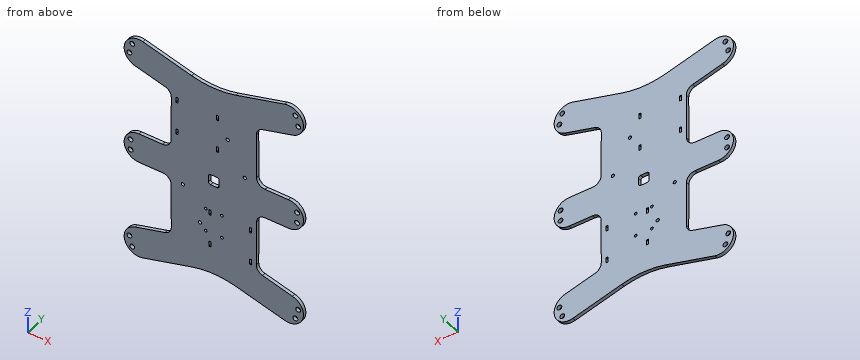
```python
from build123d import *

# Parameters (mm, degrees)
BOSS_EXTRUDE1_DEPTH = 3.175
FILLET1_R           = 80
FILLET2_R           = 8
SKETCH7_R           = 2.25
CUT_EXTRUDE4_DEPTH  = 10
CUT_EXTRUDE5_DEPTH  = 10
SKETCH9_W           = 10
SKETCH9_H           = 10
CUT_EXTRUDE6_DEPTH  = 10
FILLET3_R           = 2
SKETCH12_W          = 2
SKETCH12_H          = 5
CUT_EXTRUDE7_DEPTH  = 10
SKETCH13_R          = 1.25
CUT_EXTRUDE8_DEPTH  = 10


with BuildPart() as part:
    # Sketch1 → Boss-Extrude1 (new body)
    with BuildSketch(Plane(origin=(0, 0, 0), x_dir=(1, 0, 0), z_dir=(0, 1, 0))):
        with BuildLine():
            Line((-70, 14), (-40, 14))
            Line((-40, 14), (-39.816062711, 70))
            Line((-39.816062711, 70), (-73.623466631, 79.058666579))
            ThreePointArc((-73.623466631, 79.058666579), (-83.522961568, 96.205094778), (-66.376533369, 106.104589715))
            Line((-66.376533369, 106.104589715), (0, 88.319051202))
            Line((0, 88.319051202), (66.376533369, 106.104589715))
            ThreePointArc((66.376533369, 106.104589715), (83.522961568, 96.205094778), (73.623466631, 79.058666579))
            Line((73.623466631, 79.058666579), (39.816062711, 70))
            Line((39.816062711, 70), (40, 14))
            Line((40, 14), (70, 14))
            ThreePointArc((70, 14), (84, 0), (70, -14))
            Line((70, -14), (40, -14))
            Line((40, -14), (39.816062711, -70))
            Line((39.816062711, -70), (73.623466631, -79.058666579))
            ThreePointArc((73.623466631, -79.058666579), (83.522961568, -96.205094778), (66.376533369, -106.104589715))
            Line((66.376533369, -106.104589715), (0, -88.319051202))
            Line((0, -88.319051202), (-66.376533369, -106.104589715))
            ThreePointArc((-66.376533369, -106.104589715), (-83.522961568, -96.205094778), (-73.623466631, -79.058666579))
            Line((-73.623466631, -79.058666579), (-39.816062711, -70))
            Line((-39.816062711, -70), (-40, -14))
            Line((-40, -14), (-70, -14))
            ThreePointArc((-70, -14), (-84, 0), (-70, 14))
        make_face()
    extrude(amount=BOSS_EXTRUDE1_DEPTH)

    # Fillet1
    fillet1_edges = [part.edges().sort_by_distance(p)[0] for p in [
        (0, 1.5875, -88.319051202),
        (0, 1.5875, 88.319051202),
    ]]
    fillet(fillet1_edges, radius=FILLET1_R)

    # Fillet2
    fillet2_edges = [part.edges().sort_by_distance(p)[0] for p in [
        (-40, 1.5875, -14),
        (-39.816062711, 1.5875, -70),
        (39.816062711, 1.5875, -70),
        (40, 1.5875, -14),
        (40, 1.5875, 14),
        (39.816062711, 1.5875, 70),
        (-39.816062711, 1.5875, 70),
        (-40, 1.5875, 14),
    ]]
    fillet(fillet2_edges, radius=FILLET2_R)

    # Sketch7 → Cut-Extrude4 (cut)
    with BuildSketch(Plane(origin=(0, 3.175, 0), x_dir=(1, 0, 0), z_dir=(0, 1, 0))):
        with Locations(Location((-76.433311385, -99.481809639, 0), (0, 0, 270))):
            Circle(SKETCH7_R)
        with Locations(Location((-79.021501836, -89.822551376, 0), (0, 0, 270))):
            Circle(SKETCH7_R)
        with Locations(Location((-78, -5, 0), (0, 0, 270))):
            Circle(SKETCH7_R)
        with Locations(Location((-78, 5, 0), (0, 0, 270))):
            Circle(SKETCH7_R)
        with Locations(Location((-79.021501836, 89.822551376, 0), (0, 0, 270))):
            Circle(SKETCH7_R)
        with Locations(Location((-76.433311385, 99.481809639, 0), (0, 0, 270))):
            Circle(SKETCH7_R)
        with Locations(Location((79.021501836, 89.822551376, 0), (0, 0, 270))):
            Circle(SKETCH7_R)
        with Locations(Location((76.433311385, 99.481809639, 0), (0, 0, 270))):
            Circle(SKETCH7_R)
        with Locations(Location((78, -5, 0), (0, 0, 270))):
            Circle(SKETCH7_R)
        with Locations(Location((78, 5, 0), (0, 0, 270))):
            Circle(SKETCH7_R)
        with Locations(Location((79.021501836, -89.822551376, 0), (0, 0, 270))):
            Circle(SKETCH7_R)
        with Locations(Location((76.433311385, -99.481809639, 0), (0, 0, 270))):
            Circle(SKETCH7_R)
    extrude(amount=-CUT_EXTRUDE4_DEPTH, mode=Mode.SUBTRACT)

    # Sketch8 → Cut-Extrude5 (cut)
    with BuildSketch(Plane(origin=(0, 3.175, 0), x_dir=(1, 0, 0), z_dir=(0, 1, 0))):
        with BuildLine():
            ThreePointArc((13, -45), (11.5, -46.5), (13, -48))
            ThreePointArc((13, -48), (14.5, -46.5), (13, -45))
        make_face()
        with BuildLine():
            ThreePointArc((29, -15), (27.5, -16.5), (29, -18))
            ThreePointArc((29, -18), (30.5, -16.5), (29, -15))
        make_face()
        with BuildLine():
            ThreePointArc((-13, 48), (-14.5, 46.5), (-13, 45))
            ThreePointArc((-13, 45), (-11.5, 46.5), (-13, 48))
        make_face()
        with BuildLine():
            ThreePointArc((-29, 18), (-30.5, 16.5), (-29, 15))
            ThreePointArc((-29, 15), (-27.5, 16.5), (-29, 18))
        make_face()
    extrude(amount=-CUT_EXTRUDE5_DEPTH, mode=Mode.SUBTRACT)

    # Sketch9 → Cut-Extrude6 (cut)
    with BuildSketch(Plane(origin=(0, 3.175, 0), x_dir=(1, 0, 0), z_dir=(0, 1, 0))):
        Rectangle(SKETCH9_W, SKETCH9_H)
    extrude(amount=-CUT_EXTRUDE6_DEPTH, mode=Mode.SUBTRACT)

    # Fillet3
    fillet3_edges = [part.edges().sort_by_distance(p)[0] for p in [
        (-5, 1.5875, 5),
        (-5, 1.5875, -5),
        (5, 1.5875, -5),
        (5, 1.5875, 5),
    ]]
    fillet(fillet3_edges, radius=FILLET3_R)

    # Sketch12 → Cut-Extrude7 (cut)
    with BuildSketch(Plane(origin=(0, 3.175, 0), x_dir=(1, 0, 0), z_dir=(0, 1, 0))):
        with Locations((-34.5, -32.5)):
            Rectangle(SKETCH12_W, SKETCH12_H)
        with Locations((-34.5, -63.5)):
            Rectangle(SKETCH12_W, SKETCH12_H)
        with Locations((3.5, -63.5)):
            Rectangle(SKETCH12_W, SKETCH12_H)
        with Locations((3.5, -32.5)):
            Rectangle(SKETCH12_W, SKETCH12_H)
        with Locations((-3.5, 63.5)):
            Rectangle(SKETCH12_W, SKETCH12_H)
        with Locations((-3.5, 32.5)):
            Rectangle(SKETCH12_W, SKETCH12_H)
        with Locations((34.5, 32.5)):
            Rectangle(SKETCH12_W, SKETCH12_H)
        with Locations((34.5, 63.5)):
            Rectangle(SKETCH12_W, SKETCH12_H)
    extrude(amount=-CUT_EXTRUDE7_DEPTH, mode=Mode.SUBTRACT)

    # Sketch13 → Cut-Extrude8 (cut)
    with BuildSketch(Plane(origin=(0, 3.175, 0), x_dir=(1, 0, 0), z_dir=(0, 1, 0))):
        with Locations(Location((-7.62, 30.54, 0), (0, 0, 270))):
            Circle(SKETCH13_R)
        with Locations(Location((-7.62, 52.13, 0), (0, 0, 270))):
            Circle(SKETCH13_R)
        with Locations(Location((7.62, 52.13, 0), (0, 0, 270))):
            Circle(SKETCH13_R)
        with Locations(Location((7.62, 30.54, 0), (0, 0, 270))):
            Circle(SKETCH13_R)
    extrude(amount=-CUT_EXTRUDE8_DEPTH, mode=Mode.SUBTRACT)


solid = part.part
```
Verification items for the finished model (mm, model axes). Round coordinates to 2 decimals unless told otherwise and drop trailing zeros. Order: outer loops, then holes, each group sorted by start corner. A loop starts at its lowest first (then second) coordinate and runs counter-clockwise, first axis right, second up. Notation, with made-up numbers: (-30.75, 53.25) - (-2.75, 53.25) arc R30 ccw to (-2.75, 87.25) - close; hole circle Ø11 at (52.5, 65). An arc over 180 degrees is marked (long way). Use CSV: the item, a comma, the result in double quotes.
(1) Thickness scan on probe 1 along Z at (x, y) = (-71.5, 1.9); probe 2 along X at (y, z) = (0.3, -89.5); probe 3 along Z at (x, y) = (42.5, 1). Record the ranges inside material, lowest first. Write a range as from..to.
Entries:
probe 1,"-106.5..-78.49, -13.92..13.92, 78.49..106.5"
probe 2,"-83.66..-81.25, -76.79..76.79, 81.25..83.66"
probe 3,"-99.71..-69.83, -16.17..16.17, 69.83..99.71"
(2) Section check A-A on z = 0. Record the boundary of the cut face in (x, y) (3 decimals), and give its area (3 significant figures).
Entries:
outline,"(-84, 0) - (-5, 0) - (-5, 3.175) - (-84, 3.175) - close; (5, 0) - (84, 0) - (84, 3.175) - (5, 3.175) - close"
area,"502 mm^2"
(3) Section check C-C on y = 2.4. State how many separate pieces and enclosed holes the cut face has, and give its area (3 significant figures).
Entries:
separate pieces,"1"
enclosed holes,"29"
area,"21,700 mm^2"
(4) Gauge pin test, flat ends, axial feed: pin 1 Ø1 at (x, y) = (34.5, 2) entering from -Z; pin 2 Ø0.6 at (x, y) = (-34.5, 2) entering from -Z; pin 3 Ø1.6 at (x, y) = (-34.5, 1) entering from +Z; pin 4 Ø3 at (x, z) = (-10, 28) entering from -Y. Record the tip position at first contact, or that the pin passes through.
Entries:
pin 1,"z = -97.7"
pin 2,"z = -97.64"
pin 3,"z = 97.78"
pin 4,"y = 0"
(5) Section check D-D on z = -84. Record the boundary of the cut face in (x, y) (3 decimals).
Entries:
outline,"(-81.061, 0) - (81.061, 0) - (81.061, 3.175) - (-81.061, 3.175) - close"
(6) Section check B-B on x = 51.5. Record the boundary of the cut face in (y, z) (3 decimals), and give its area (3 significant figures).
Entries:
outline,"(0, -102.118) - (3.175, -102.118) - (3.175, -73.131) - (0, -73.131) - close; (0, -14) - (3.175, -14) - (3.175, 14) - (0, 14) - close; (0, 73.131) - (3.175, 73.131) - (3.175, 102.118) - (0, 102.118) - close"
area,"273 mm^2"
